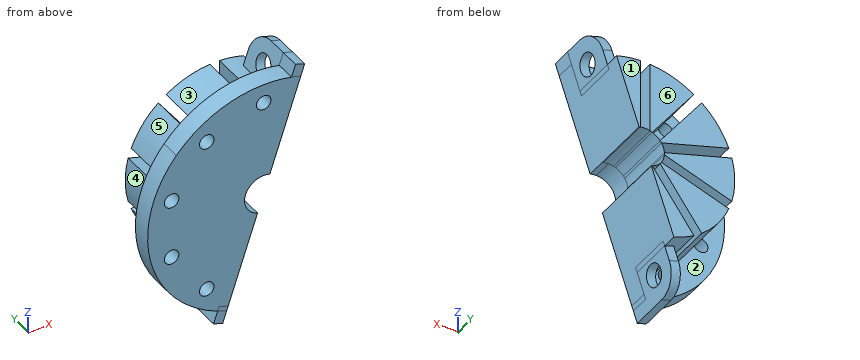
```python
from build123d import *
from build123d.topology import SkipClean

# Parameters (mm, degrees)
SKETCH1_R           = 11.984375
SKETCH1_R_2         = 1.984375
SKETCH1_R_3         = 0.75
BOSS_EXTRUDE1_DEPTH = 2
SKETCH6_W           = 23.96875
SKETCH6_H           = 8
CUT_EXTRUDE1_DEPTH  = 19.741677841
BOSS_EXTRUDE3_START = -2
SKETCH7_R           = 1.65
BOSS_EXTRUDE3_DEPTH = 2
SKETCH8_R           = 1.1
BOSS_EXTRUDE4_DEPTH = 1
CUT_EXTRUDE2_DEPTH  = 23.122053344


with BuildPart() as part:
    # Sketch1 → Boss-Extrude1 (new body)
    with BuildSketch(Plane(origin=(0, 0, 0), x_dir=(1, 0, 0), z_dir=(0, 1, 0))):
        with Locations(Location((0, 0, 0), (0, 0, 270))):
            Circle(SKETCH1_R)
        with Locations(Location((0, 0, 0), (0, 0, 270))):
            Circle(SKETCH1_R_2, mode=Mode.SUBTRACT)
        with Locations(Location((0, 10, 0), (0, 0, 270))):
            Circle(SKETCH1_R_3, mode=Mode.SUBTRACT)
        with Locations(Location((5.877852523, 8.090169944, 0), (0, 0, 270))):
            Circle(SKETCH1_R_3, mode=Mode.SUBTRACT)
        with Locations(Location((9.510565163, 3.090169944, 0), (0, 0, 270))):
            Circle(SKETCH1_R_3, mode=Mode.SUBTRACT)
        with Locations(Location((9.510565163, -3.090169944, 0), (0, 0, 270))):
            Circle(SKETCH1_R_3, mode=Mode.SUBTRACT)
        with Locations(Location((5.877852523, -8.090169944, 0), (0, 0, 270))):
            Circle(SKETCH1_R_3, mode=Mode.SUBTRACT)
        with Locations(Location((0, -10, 0), (0, 0, 270))):
            Circle(SKETCH1_R_3, mode=Mode.SUBTRACT)
        with Locations(Location((-5.877852523, -8.090169944, 0), (0, 0, 270))):
            Circle(SKETCH1_R_3, mode=Mode.SUBTRACT)
        with Locations(Location((-9.510565163, -3.090169944, 0), (0, 0, 270))):
            Circle(SKETCH1_R_3, mode=Mode.SUBTRACT)
        with Locations(Location((-9.510565163, 3.090169944, 0), (0, 0, 270))):
            Circle(SKETCH1_R_3, mode=Mode.SUBTRACT)
        with Locations(Location((-5.877852523, 8.090169944, 0), (0, 0, 270))):
            Circle(SKETCH1_R_3, mode=Mode.SUBTRACT)
    extrude(amount=BOSS_EXTRUDE1_DEPTH)

    # Sweep1: sweep along a path in Sketch3
    with SkipClean():  # the faces are left unmerged after this step: merging them gives an invalid solid
        with BuildLine(Plane(origin=(0, 0, 0), x_dir=(0, 0, -1), z_dir=(1, 0, 0))) as sweep1_path:
            Line((0, 2), (0, 8))
        # Sketch2 → Sweep1 (sweep)
        with BuildSketch(Plane(origin=(0, 2, 0), x_dir=(1, 0, 0), z_dir=(0, 1, 0))):
            with BuildLine():
                Line((-0.5, 9.236476601), (-0.5, 1.920350005))
                ThreePointArc((-0.5, 1.920350005), (-0.613205598, 1.887252775), (-0.724244915, 1.847488415))
                Line((-0.724244915, 1.847488415), (-5.024556232, 7.766359164))
                ThreePointArc((-5.024556232, 7.766359164), (-2.858407198, 8.797272776), (-0.5, 9.236476601))
            make_face()
            with BuildLine():
                Line((0.5, 9.236476601), (0.5, 1.920350005))
                ThreePointArc((0.5, 1.920350005), (0.613205598, 1.887252775), (0.724244915, 1.847488415))
                Line((0.724244915, 1.847488415), (5.024556232, 7.766359164))
                ThreePointArc((5.024556232, 7.766359164), (2.858407198, 8.797272776), (0.5, 9.236476601))
            make_face()
            with BuildLine():
                Line((5.833573226, 7.178573912), (1.533261909, 1.259703163))
                ThreePointArc((1.533261909, 1.259703163), (1.605393098, 1.16638636), (1.671852888, 1.068949045))
                Line((1.671852888, 1.068949045), (8.629902762, 3.329756496))
                ThreePointArc((8.629902762, 3.329756496), (7.483407198, 5.437013584), (5.833573226, 7.178573912))
            make_face()
            with BuildLine():
                Line((8.938919756, 2.37869998), (1.980869883, 0.117892528))
                ThreePointArc((1.980869883, 0.117892528), (1.984375, 0), (1.980869883, -0.117892528))
                Line((1.980869883, -0.117892528), (8.938919756, -2.37869998))
                ThreePointArc((8.938919756, -2.37869998), (9.25, 0), (8.938919756, 2.37869998))
            make_face()
            with BuildLine():
                Line((8.629902762, -3.329756496), (1.671852888, -1.068949045))
                ThreePointArc((1.671852888, -1.068949045), (1.605393098, -1.16638636), (1.533261909, -1.259703163))
                Line((1.533261909, -1.259703163), (5.833573226, -7.178573912))
                ThreePointArc((5.833573226, -7.178573912), (7.483407198, -5.437013584), (8.629902762, -3.329756496))
            make_face()
            with BuildLine():
                Line((5.024556232, -7.766359164), (0.724244915, -1.847488415))
                ThreePointArc((0.724244915, -1.847488415), (0.613205598, -1.887252775), (0.5, -1.920350005))
                Line((0.5, -1.920350005), (0.5, -9.236476601))
                ThreePointArc((0.5, -9.236476601), (2.858407198, -8.797272776), (5.024556232, -7.766359164))
            make_face()
            with BuildLine():
                Line((-0.5, -9.236476601), (-0.5, -1.920350005))
                ThreePointArc((-0.5, -1.920350005), (-0.613205598, -1.887252775), (-0.724244915, -1.847488415))
                Line((-0.724244915, -1.847488415), (-5.024556232, -7.766359164))
                ThreePointArc((-5.024556232, -7.766359164), (-2.858407198, -8.797272776), (-0.5, -9.236476601))
            make_face()
            with BuildLine():
                Line((-5.833573226, -7.178573912), (-1.533261909, -1.259703163))
                ThreePointArc((-1.533261909, -1.259703163), (-1.605393098, -1.16638636), (-1.671852888, -1.068949045))
                Line((-1.671852888, -1.068949045), (-8.629902762, -3.329756496))
                ThreePointArc((-8.629902762, -3.329756496), (-7.483407198, -5.437013584), (-5.833573226, -7.178573912))
            make_face()
            with BuildLine():
                Line((-8.938919756, -2.37869998), (-1.980869883, -0.117892528))
                ThreePointArc((-1.980869883, -0.117892528), (-1.984375, 0), (-1.980869883, 0.117892528))
                Line((-1.980869883, 0.117892528), (-8.938919756, 2.37869998))
                ThreePointArc((-8.938919756, 2.37869998), (-9.25, 0), (-8.938919756, -2.37869998))
            make_face()
            with BuildLine():
                Line((-8.629902762, 3.329756496), (-1.671852888, 1.068949045))
                ThreePointArc((-1.671852888, 1.068949045), (-1.605393098, 1.16638636), (-1.533261909, 1.259703163))
                Line((-1.533261909, 1.259703163), (-5.833573226, 7.178573912))
                ThreePointArc((-5.833573226, 7.178573912), (-7.483407198, 5.437013584), (-8.629902762, 3.329756496))
            make_face()
        sweep(path=sweep1_path.line)

    # Sketch4 → Revolve1 (revolve)
    with SkipClean():  # the faces are left unmerged after this step: merging them gives an invalid solid
        with BuildSketch(Plane(origin=(0, 0, 0), x_dir=(0, 0, -1), z_dir=(1, 0, 0)), mode=Mode.PRIVATE) as revolve1_sk:
            Polygon((-2.37869998, 2), (-1.984375, 2), (-1.984375, 8), align=None)
        revolve(revolve1_sk.sketch.rotate(Axis((0, 0, 0), (0, 1, 0)), 165.405971265), axis=Axis((0, 0, 0), (0, 1, 0)))

    # Sketch6 → Cut-Extrude1 (cut, through all)
    with SkipClean():  # the faces are left unmerged after this step: merging them gives an invalid solid
        with BuildSketch(Plane(origin=(0, 0, 0), x_dir=(-0.3193728209047868, 0, -0.9476291475399641), z_dir=(-0.9476291475399641, 0, 0.3193728209047868))):
            with Locations((0, -4)):
                Rectangle(SKETCH6_W, SKETCH6_H)
        extrude(amount=-CUT_EXTRUDE1_DEPTH, mode=Mode.SUBTRACT)

    # Sketch7 → Boss-Extrude3 (add)
    with SkipClean():  # the faces are left unmerged after this step: merging them gives an invalid solid
        with BuildSketch(Plane(origin=(0, 2, 0), x_dir=(1, 0, 0), z_dir=(0, 1, 0)).offset(BOSS_EXTRUDE3_START)):
            with BuildLine():
                Line((-9.021857716, -7.888683508), (-1.576209535, -16.403865848))
                ThreePointArc((-1.576209535, -16.403865848), (2.803074288, -17.134270389), (4.375298385, -12.982195127))
                Line((4.375298385, -12.982195127), (3.827483651, -11.356743065))
                ThreePointArc((3.827483651, -11.356743065), (-3.122857627, -11.570350227), (-9.021857716, -7.888683508))
            make_face()
            with Locations(Location((1.058596369, -14.1, 0), (0, 0, 270))):
                Circle(SKETCH7_R, mode=Mode.SUBTRACT)
        extrude(amount=BOSS_EXTRUDE3_DEPTH)

    # Sketch8 → Boss-Extrude4 (add)
    # profile 1 of 2: a face of its own
    with SkipClean():  # the faces are left unmerged after this step: merging them gives an invalid solid
        with BuildSketch(Plane(origin=(0, 0, 0), x_dir=(-0.31937282090478675, 0, -0.9476291475399641), z_dir=(0.9476291475399641, 0, -0.31937282090478675))):
            with BuildLine():
                Line((-13.25, 4), (-13.25, 2))
                Line((-13.25, 2), (-8.75, 2))
                Line((-8.75, 2), (-8.75, 6.5))
                Line((-8.75, 6.5), (-9.25, 6.5))
                Line((-9.25, 6.5), (-10.75, 6.5))
                ThreePointArc((-10.75, 6.5), (-12.517766953, 5.767766953), (-13.25, 4))
            make_face()
            with Locations((-10.75, 4)):
                Circle(SKETCH8_R, mode=Mode.SUBTRACT)
        # profile 2 of 2: a face of its own
        with BuildSketch(Plane(origin=(0, 0, 0), x_dir=(-0.31937282090478675, 0, -0.9476291475399641), z_dir=(0.9476291475399641, 0, -0.31937282090478675))):
            with BuildLine():
                Line((11.484375, 2), (8.75, 2))
                Line((8.75, 2), (8.75, 6.5))
                Line((8.75, 6.5), (9.25, 6.5))
                Line((9.25, 6.5), (10.75, 6.5))
                ThreePointArc((10.75, 6.5), (12.517766953, 5.767766953), (13.25, 4))
                Line((13.25, 4), (13.25, 2))
                Line((13.25, 2), (13.25, 0))
                Line((13.25, 0), (11.984375, 0))
                Line((11.984375, 0), (11.484375, 0))
                Line((11.484375, 0), (11.484375, 2))
            make_face()
            with Locations((10.75, 4)):
                Circle(SKETCH8_R, mode=Mode.SUBTRACT)
        extrude(amount=-BOSS_EXTRUDE4_DEPTH)

    # Sketch9 → Cut-Extrude2 (cut, through all)
    with SkipClean():  # the faces are left unmerged after this step: merging them gives an invalid solid
        with BuildSketch(Plane(origin=(0, 2, 0), x_dir=(1, 0, 0), z_dir=(0, 1, 0))):
            with BuildLine():
                Line((-9.021857716, -7.888683508), (-1.576209535, -16.403865848))
                ThreePointArc((-1.576209535, -16.403865848), (2.803074288, -17.134270389), (4.375298385, -12.982195127))
                Line((4.375298385, -12.982195127), (4.231689877, -12.556086205))
                Line((4.231689877, -12.556086205), (3.284060729, -12.875459026))
                Line((3.284060729, -12.875459026), (2.866506678, -11.6365108))
                ThreePointArc((2.866506678, -11.6365108), (-3.603281692, -11.429855869), (-9.021857716, -7.888683508))
            make_face()
        extrude(amount=-CUT_EXTRUDE2_DEPTH, mode=Mode.SUBTRACT)


solid = part.part
```
Read the model definition and answer for the solid it produces. Units are mm, in the model's axes. Face numbers are marked on the shaded views. A direction names the side the tool comes from. Coordinates: 2 decimals unless noted, no trailing zeros. Loops run counter-clockwise (first coordinate to the right, second up) from the corner with the lowest first, then second, coordinate; pieces in that order, holes last. Notation, with made-up numbers: (34, 28) - (87, 28) arc R23 cw to (87, 55) - close; hole circle Ø3 at (78, 16). An arc over 180 degrees is marked (long way). Answer in a Markdown table with one row per item.
1. Given pin 1 (4 mm diameter, centred on x = -9, z = 4.5, fed in from -Y); pin 2 (1.8 mm diameter, centred on y = 5, z = 6, fed in from -X); pin 3 (1.7 mm diameter, centred on x = -9.51, z = 3.09, fed in from +Y); pin 4 (0.7 mm diameter, centred on x = 3, z = 9.5, fed in from +Y), each flat-ended and moving along its own axis, determine where each tip first touches the part or whether it passes through.
Conclusion:
| item | result |
|---|---|
| pin 1 | stops at y = 0 |
| pin 2 | stops at x = -7.72 |
| pin 3 | stops at y = 2 |
| pin 4 | stops at y = 6.5 |
2. Straight lines are drawn through the part: line 1 (Z direction, x = -9, y = 1); line 2 (Z direction, x = -4.5, y = 7.25); line 3 (Z direction, x = 0.5, y = 1.5). For each, find the intervals that lie inside material, in ascending order.
Conclusion:
| item | result |
|---|---|
| line 1 | z = -7.91 to -3.64, -2.54 to 2.54, 3.64 to 7.91 |
| line 2 | z = -8.08 to -7.04, -5.34 to -1.99, -0.94 to 0.94, 1.99 to 5.34, 7.04 to 8.08 |
| line 3 | z = 1.92 to 9.44, 10.56 to 11.97 |
3. Find section D-D, the plane x = 1.25. Write down the section's boundary in (y, z).
Conclusion:
| item | result |
|---|---|
| outline | (0, 3.71) - (8, 3.71) - (8, 9.17) - (2, 9.17) - (2, 11.92) - (0, 11.92) - close |
4. Which of the six approach directions +Z, -Z, +X, -X, +Y, -Y give full straight-line access (tool end or side, diameter ignored) to the marked faces 4, 5 and 6?
Conclusion:
| item | result |
|---|---|
| face 4 | -X, +Y |
| face 5 | +Z, -X, +Y |
| face 6 | +Z, -Z, +X, -X, +Y |
5. Determine the mould class of the marked faces 1, 2 and 3 for opening direction Z: +Z half, -Z half, draft (parallel to the pull), parting line (faces both ways), or undercut.
Conclusion:
| item | result |
|---|---|
| face 1 | draft |
| face 2 | undercut |
| face 3 | +Z half |
6. Find section B-B, the plane z = 4.25. Write down the section's boundary in (x, y).
Conclusion:
| item | result |
|---|---|
| outline | (-11.21, 0) - (1.43, 0) - (1.43, 8) - (0.5, 8) - (0.5, 2) - (-0.5, 2) - (-0.5, 8) - (-2.47, 8) - (-2.47, 2) - (-3.71, 2) - (-3.71, 8) - (-8.22, 8) - (-8.22, 2) - (-11.21, 2) - close |
7. Find section C-C, the plane y = 7.5. Write down the section's boundary in (x, z), then the cut area to 3 significant figures.
Conclusion:
| item | result |
|---|---|
| outline | (-8.94, -2.38) - (-2.01, -0.13) arc R2.02 ccw to (-1.7, -1.08) - (-8.63, -3.33) arc R9.25 ccw to (-5.83, -7.18) - (-1.55, -1.29) arc R2.02 ccw to (-0.74, -1.87) - (-5.02, -7.77) arc R9.25 ccw to (-2.95, -8.77) - (-0.63, -1.88) arc R1.98 cw to (0.63, 1.88) - (2.95, 8.77) arc R9.25 ccw to (0.5, 9.24) - (0.5, 1.95) arc R2.02 ccw to (-0.5, 1.95) - (-0.5, 9.24) arc R9.25 ccw to (-5.02, 7.77) - (-0.74, 1.87) arc R2.02 ccw to (-1.55, 1.29) - (-5.83, 7.18) arc R9.25 ccw to (-8.63, 3.33) - (-1.7, 1.08) arc R2.02 ccw to (-2.01, 0.13) - (-8.94, 2.38) arc R9.25 ccw to start |
| area | 92.0 mm² |
